Work out the finished part from the listing and answer in its coordinate system (mm). A direction names the side the tool comes from. Round coordinates to 2 decimals unless told otherwise and drop trailing zeros. Write each loop counter-clockwise with the first axis right and the second up, starting at its lowest first coordinate (ties: lowest second). Pieces come first, ordered by that corner, then holes. Notation, with made-up numbers: (27.5, 41.5) - (42.5, 41.5) arc R36 cw to (42.5, 77.5) - close; hole circle Ø7 at (14, 82.25). An arc over 180 degrees is marked (long way). Answer as a JSON object with one key per item and string values.
```python
from build123d import *

# Parameters (mm, degrees)
IZIM1_R                     = 2.55
IZIM1_R_2                   = 3
IZIM1_R_3                   = 6.5
IZIM1_R_4                   = 1.7
Y_KSEKLIK_EKSTR_ZYON1_DEPTH = 4.4
IZIM2_R                     = 19
IZIM2_R_2                   = 6.5
Y_KSEKLIK_EKSTR_ZYON2_DEPTH = 1.5
PAH1_SIZE                   = 0.2
PAH2_SIZE                   = 0.75
KES_EKSTR_ZYON1_START       = -3
IZIM3_R                     = 3.125
IZIM3_R_2                   = 1.7
IZIM3_R_3                   = 2.75
KES_EKSTR_ZYON1_DEPTH       = 3
PAH3_SIZE                   = 0.2
IZIM4_R                     = 11
KES_EKSTR_ZYON2_DEPTH       = 3.66
IZIM5_R                     = 8.9
KES_EKSTR_ZYON3_DEPTH       = 0.5
PAH4_SIZE                   = 0.2
Y_KSEKLIK_EKSTR_ZYON3_START = 2.9
IZIM6_R                     = 12.75
IZIM6_R_2                   = 11
Y_KSEKLIK_EKSTR_ZYON3_DEPTH = 2.9
PAH5_SIZE                   = 0.2
PAH5_SIZE2                  = 0.746410162
IZIM7_R                     = 28.3
IZIM7_R_2                   = 26.75
Y_KSEKLIK_EKSTR_ZYON4_DEPTH = 10.06
KES_EKSTR_ZYON4_START       = -0.5
IZIM8_R                     = 12.75
KES_EKSTR_ZYON4_DEPTH       = 0.5
IZIM10_R                    = 27.5
KES_EKSTR_ZYON5_DEPTH       = 1.5


with BuildPart() as part:
    # Çizim1 → Yükseklik-Ekstrüzyon1 (new body)
    with BuildSketch(Plane.XY):
        with BuildLine():
            Line((-23.85, 28.3), (23.85, 28.3))
            ThreePointArc((23.85, 28.3), (26.996625176, 26.996625176), (28.3, 23.85))
            Line((28.3, 23.85), (28.3, -23.85))
            ThreePointArc((28.3, -23.85), (26.996625176, -26.996625176), (23.85, -28.3))
            Line((23.85, -28.3), (-23.85, -28.3))
            ThreePointArc((-23.85, -28.3), (-26.996625176, -26.996625176), (-28.3, -23.85))
            Line((-28.3, -23.85), (-28.3, 23.85))
            ThreePointArc((-28.3, 23.85), (-26.996625176, 26.996625176), (-23.85, 28.3))
        make_face()
        with Locations((-23.511300474, 23.511300474)):
            Circle(IZIM1_R, mode=Mode.SUBTRACT)
        with Locations((23.511300474, -23.511300474)):
            Circle(IZIM1_R, mode=Mode.SUBTRACT)
        with Locations((-23.511300474, -23.511300474)):
            Circle(IZIM1_R_2, mode=Mode.SUBTRACT)
        with Locations((23.511300474, 23.511300474)):
            Circle(IZIM1_R_2, mode=Mode.SUBTRACT)
        Circle(IZIM1_R_3, mode=Mode.SUBTRACT)
        with Locations((0, 25)):
            Circle(IZIM1_R_4, mode=Mode.SUBTRACT)
        with Locations((21.650635095, -12.5)):
            Circle(IZIM1_R_4, mode=Mode.SUBTRACT)
        with Locations((-21.650635095, -12.5)):
            Circle(IZIM1_R_4, mode=Mode.SUBTRACT)
    extrude(amount=Y_KSEKLIK_EKSTR_ZYON1_DEPTH)

    # Çizim2 → Yükseklik-Ekstrüzyon2 (add)
    with BuildSketch(Plane.XY.offset(4.4)):
        with Locations(Location((0, 0, 0), (0, 0, 180))):
            Circle(IZIM2_R)
        Circle(IZIM2_R_2, mode=Mode.SUBTRACT)
    extrude(amount=Y_KSEKLIK_EKSTR_ZYON2_DEPTH)

    # Pah1
    pah1_edges = [part.edges().sort_by_distance(p)[0] for p in [
        (19, 0, 5.9),
    ]]
    chamfer(pah1_edges, length=PAH1_SIZE)

    # Pah2
    pah2_edges = [part.edges().sort_by_distance(p)[0] for p in [
        (20.511300474, 23.511300474, 4.4),
        (-26.511300474, -23.511300474, 4.4),
    ]]
    chamfer(pah2_edges, length=PAH2_SIZE)

    # Çizim3 → Kes-Ekstrüzyon1 (cut)
    # profile 1 of 3: a face of its own
    with BuildSketch(Plane.XY.offset(4.4).offset(KES_EKSTR_ZYON1_START)):
        with Locations((-21.650635095, -12.5)):
            Circle(IZIM3_R)
        with Locations((-21.650635095, -12.5)):
            Circle(IZIM3_R_2, mode=Mode.SUBTRACT)
    # profile 2 of 3: a face of its own
    with BuildSketch(Plane.XY.offset(4.4).offset(KES_EKSTR_ZYON1_START)):
        with Locations((21.650635095, -12.5)):
            Circle(IZIM3_R)
        with Locations((21.650635095, -12.5)):
            Circle(IZIM3_R_2, mode=Mode.SUBTRACT)
    # profile 3 of 3: a face of its own
    with BuildSketch(Plane.XY.offset(4.4).offset(KES_EKSTR_ZYON1_START)):
        with Locations((0, 25)):
            Circle(IZIM3_R_3)
        with Locations((0, 25)):
            Circle(IZIM3_R_2, mode=Mode.SUBTRACT)
    extrude(amount=KES_EKSTR_ZYON1_DEPTH, mode=Mode.SUBTRACT)

    # Pah3
    pah3_edges = [part.edges().sort_by_distance(p)[0] for p in [
        (-26.061300474, 23.511300474, 4.4),
        (20.961300474, -23.511300474, 4.4),
        (-24.775635095, -12.5, 4.4),
        (18.525635095, -12.5, 4.4),
        (-2.75, 25, 4.4),
    ]]
    chamfer(pah3_edges, length=PAH3_SIZE)

    # Çizim4 → Kes-Ekstrüzyon2 (cut)
    with BuildSketch(Plane(origin=(0, 0, 0), x_dir=(-1, 0, 0), z_dir=(0, 0, -1))):
        Circle(IZIM4_R)
    extrude(amount=-KES_EKSTR_ZYON2_DEPTH, mode=Mode.SUBTRACT)

    # Çizim5 → Kes-Ekstrüzyon3 (cut)
    with BuildSketch(Plane(origin=(0, 0, 3.66), x_dir=(-1, 0, 0), z_dir=(0, 0, -1))):
        Circle(IZIM5_R)
    extrude(amount=-KES_EKSTR_ZYON3_DEPTH, mode=Mode.SUBTRACT)

    # Pah4
    pah4_edges = [part.edges().sort_by_distance(p)[0] for p in [
        (-6.5, 0, 4.16),
    ]]
    chamfer(pah4_edges, length=PAH4_SIZE)

    # Çizim6 → Yükseklik-Ekstrüzyon3 (add)
    with BuildSketch(Plane(origin=(0, 0, 0), x_dir=(-1, 0, 0), z_dir=(0, 0, -1)).offset(Y_KSEKLIK_EKSTR_ZYON3_START)):
        Circle(IZIM6_R)
        Circle(IZIM6_R_2, mode=Mode.SUBTRACT)
    extrude(amount=-Y_KSEKLIK_EKSTR_ZYON3_DEPTH)

    # Pah5
    pah5_edges = [part.edges().sort_by_distance(p)[0] for p in [
        (11, 0, -2.9),
    ]]
    pah5_side = [part.faces().sort_by_distance(p)[0] for p in [
        (12.389375542, 0, -2.9),
    ]]
    chamfer(pah5_edges, length=PAH5_SIZE, length2=PAH5_SIZE2, reference=pah5_side[0])

    # Çizim7 → Yükseklik-Ekstrüzyon4 (add)
    with BuildSketch(Plane(origin=(0, 0, 0), x_dir=(-1, 0, 0), z_dir=(0, 0, -1))):
        Circle(IZIM7_R)
        Circle(IZIM7_R_2, mode=Mode.SUBTRACT)
    extrude(amount=Y_KSEKLIK_EKSTR_ZYON4_DEPTH)

    # Çizim8 → Kes-Ekstrüzyon4 (cut)
    with BuildSketch(Plane(origin=(0, 0, 0), x_dir=(-1, 0, 0), z_dir=(0, 0, -1)).offset(KES_EKSTR_ZYON4_START)):
        with BuildLine():
            Line((-2.9, 25), (-2.9, 26.592339122))
            ThreePointArc((-2.9, 26.592339122), (-23.166179551, 13.375), (-24.479641226, -10.78469589))
            Line((-24.479641226, -10.78469589), (-23.100635095, -9.988526329))
            ThreePointArc((-23.100635095, -9.988526329), (-19.139161424, -11.05), (-20.200635095, -15.011473671))
            Line((-20.200635095, -15.011473671), (-21.579641226, -15.807643232))
            ThreePointArc((-21.579641226, -15.807643232), (0, -26.75), (21.579641226, -15.807643232))
            Line((21.579641226, -15.807643232), (20.200635095, -15.011473671))
            ThreePointArc((20.200635095, -15.011473671), (19.139161424, -11.05), (23.100635095, -9.988526329))
            Line((23.100635095, -9.988526329), (24.479641226, -10.78469589))
            ThreePointArc((24.479641226, -10.78469589), (23.166179551, 13.375), (2.9, 26.592339122))
            Line((2.9, 26.592339122), (2.9, 25))
            ThreePointArc((2.9, 25), (0, 22.1), (-2.9, 25))
        make_face()
        Circle(IZIM8_R, mode=Mode.SUBTRACT)
    extrude(amount=KES_EKSTR_ZYON4_DEPTH, mode=Mode.SUBTRACT)

    # Çizim10 → Kes-Ekstrüzyon5 (cut)
    with BuildSketch(Plane(origin=(0, 0, -10.06), x_dir=(-1, 0, 0), z_dir=(0, 0, -1))):
        Circle(IZIM10_R)
    extrude(amount=-KES_EKSTR_ZYON5_DEPTH, mode=Mode.SUBTRACT)


solid = part.part
```
Item 1: A cutting plane is placed at A-A (z = -1.25). Write down the section's boundary in (x, y).
Results found:
{"outline": "circle Ø56.6 at (0, 0); circle Ø25.5 at (0, 0); hole circle Ø53.5 at (0, 0); hole circle Ø22 at (0, 0)"}
Item 2: For faces 1 (the cylindrical face through (5.961, -26.846, -9.32)), 2 (the cylindrical face through (-24.773, -12.363, 2.78)), 3 (the flat face through (0, 28.3, 2)), determine the directions among +Z, -Z, +X, -X, +Y, -Y from which every point of the face is accessible in a straight line to the end or side of a thin tool.
Results found:
{"face 1": "-Z", "face 2": "+Z", "face 3": "+Z, -Z, +X, -X, +Y"}
Item 3: Determine the mould class of faces 4 (the flat face through (0, 8, 5.9)), 5 (the cylindrical face through (-23.35, -12.43, 0.69)), 6 (the cylindrical face through (26.962, 27.031, 2.169)) for opening direction Y: pulls with the +Y half, pulls with the -Y half, needs draft (parallel to the pull), parting line crosses it, or undercut.
Results found:
{"face 4": "needs draft", "face 5": "undercut", "face 6": "pulls with the +Y half"}
Item 4: Consider line 1 along Y through (x, z) = (0, 3.9); line 2 along Y through (x, z) = (-1.5, 2.25); line 3 along Z through (x, y) = (13, -5). Determine where each line is inside the solid, lowest interval first.
Results found:
{"line 1": "-28.3 to -8.9, 8.9 to 22.25, 27.75 to 28.3", "line 2": "-28.3 to -10.9, 10.9 to 22.7, 27.3 to 28.3", "line 3": "0.5 to 5.9"}
Item 5: Each of these flat-tipped pins is pushed along its axis until it touches: P1, Ø4, axis at y = 8, z = -8, coming from the -X side; P2, Ø16, axis at x = -3, y = 2.5, coming from the -Z side; P3, Ø6.5, axis at x = 4.5, y = -3, coming from the -Z side. Where does it stop, or does it pass through?
Results found:
{"P1": "x = -27.66", "P2": "z = -2.9", "P3": "z = 4.16"}
